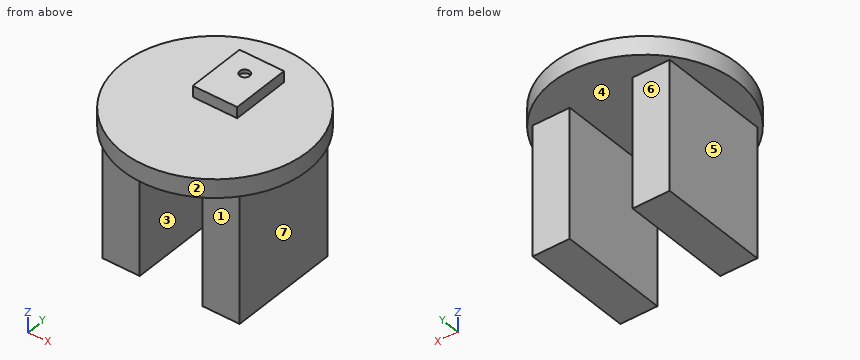
```python
from build123d import *

# Parameters (mm, degrees)
F0_R     = 6.35
F1_DEPTH = 1.27
F2_W     = 3.048
F2_H     = 4.064
F3_DEPTH = 0.762
F4_R     = 0.34925
F5_DEPTH = 0.254
F6_W     = 2.54
F6_H     = 7.62
F7_DEPTH = 8.89


with BuildPart() as f1:
    # F0 (on Top) → F1 (new body)
    with BuildSketch(Plane.XY):
        Circle(F0_R)
    extrude(amount=F1_DEPTH)

    # F2 (on face) → F3 (join)
    with BuildSketch(Plane.XY.offset(1.27)):
        with Locations((0, 2.032)):
            Rectangle(F2_W, F2_H)
    extrude(amount=F3_DEPTH)

    # F4 (on face) → F5 (cut)
    with BuildSketch(Plane.XY.offset(2.032)):
        with Locations((0, 2.5908)):
            Circle(F4_R)
    extrude(amount=-F5_DEPTH, mode=Mode.SUBTRACT)

    # F6 (on face) → F7 (join)
    with BuildSketch(Plane(origin=(0, 0, 0), x_dir=(1, 0, 0), z_dir=(0, 0, -1))):
        with Locations((-3.429, 0)):
            Rectangle(F6_W, F6_H)
    extrude(amount=F7_DEPTH)

    # F8: F1 across plane


with BuildPart() as f1_1:
    add(f1.part)
    add(f1.part.mirror(Plane.YZ))


solid = f1_1.part
```
Can you work these out from the model? Positions are in its coordinate system, mm. Face numbers are marked on the shaded views. A direction names the side the tool comes from. Give positions to 0.01 mm unless a question says otherwise; leave off trailing zeros. Order: outer loops, then holes, each group sorted by start corner. A loop starts at its lowest first (then second) coordinate and runs counter-clockwise, first axis right, second up. Notation, with made-up numbers: M 16,61.5 L 64,61.5 A31 cw 64,99.5 Z; hole C -31,31.5 d1. An arc over 180 degrees is marked long. One line per item, written item: value.
1) I want a section at D-D, the plane x = 4. List the corners of the cut face in (y, z) for me.
Answer sheet:
outline: M -4.93,0 L -3.81,0 L -3.81,-8.89 L 3.81,-8.89 L 3.81,0 L 4.93,0 L 4.93,1.27 L -4.93,1.27 Z
2) I want a section at C-C, the plane y = 1.25. List the corners of the cut face in (x, z) for me, plus the area to 3 significant figures.
Answer sheet:
outline: M -6.23,0 L -4.7,0 L -4.7,-8.89 L -2.16,-8.89 L -2.16,0 L 2.16,0 L 2.16,-8.89 L 4.7,-8.89 L 4.7,0 L 6.23,0 L 6.23,1.27 L 1.52,1.27 L 1.52,2.03 L -1.52,2.03 L -1.52,1.27 L -6.23,1.27 Z
area: 63.3 mm^2
3) For P1, Ø1, axis at y = 0, z = -6.5, coming from the +X side; P2, Ø2.5, axis at y = -0.5, z = -6.5, coming from the -X side; P3, Ø3, axis at x = -3.5, z = -3.5, coming from the +Y side, each with a flat end and sliding along its axis, tell me the tip position at first contact or that it passes through.
Answer sheet:
P1: stops at x = 4.7
P2: stops at x = -4.7
P3: stops at y = 3.81
4) Please list where these lines run through material, in increasing order: line 1 along X through (y, z) = (-1, -6.75); line 2 along Y through (x, z) = (0, 1.95); line 3 along Z through (x, y) = (-0.25, 5).
Answer sheet:
line 1: x = -4.7 to -2.16, 2.16 to 4.7
line 2: y = 0 to 2.24, 2.94 to 4.06
line 3: z = 0 to 1.27
5) We'd pull the mould along X, two halves only. Please class the marked faces 1, 2, 3 and 4: released by +X, released by -X, zero draft, split by the parting line, or undercut.
Answer sheet:
face 1: zero draft
face 2: split by the parting line
face 3: undercut
face 4: undercut
6) I want a section at A-A, the plane z = -2.75. List the corners of the cut face in (x, y) for me.
Answer sheet:
outline: M -4.7,-3.81 L -2.16,-3.81 L -2.16,3.81 L -4.7,3.81 Z; M 2.16,-3.81 L 4.7,-3.81 L 4.7,3.81 L 2.16,3.81 Z
7) On a 3-axis mill with a long thin cutter (end or side, diameter ignored), from which of +Z, -Z, +X, -X, +Y, -Y can I reach the whole of each face in a straight line? I mean the marked faces 5, 6 and 7. Say none if no direction works.
Answer sheet:
face 5: -Z, -X, +Y, -Y
face 6: -Z, +X, -X, +Y
face 7: -Z, +X, +Y, -Y
8) I want a section at B-B, the plane x = 0. List the corners of the cut face in (y, z) for me.
Answer sheet:
outline: M -6.35,0 L 6.35,0 L 6.35,1.27 L 4.06,1.27 L 4.06,2.03 L 2.94,2.03 L 2.94,1.78 L 2.24,1.78 L 2.24,2.03 L 0,2.03 L 0,1.27 L -6.35,1.27 Z
